Model file for the job. Use its own axes, mm. A direction names the side the tool comes from. Give positions to 0.01 mm unless a question says otherwise; leave off trailing zeros. Write each loop counter-clockwise with the first axis right and the second up, starting at its lowest first coordinate (ties: lowest second). Pieces come first, ordered by that corner, then holes.
```python
from build123d import *

# Parameters (mm, degrees)
EXTRUDE1_DEPTH          = 15.875
SKETCH2_W               = 56.3626
SKETCH2_H               = 56.3626
CUT_EXTRUDE1_DEPTH      = 3.9624
SKETCH3_W               = 56.3626
SKETCH3_H               = 56.3626
CUT_EXTRUDE2_DEPTH      = 3.9624
CUT_EXTRUDE3_DEPTH      = 174.221342401
CUT_EXTRUDE4_DEPTH      = 138.612224622
SKETCH7_R               = 3.175
CUT_EXTRUDE6_DEPTH      = 174.221342401
CUT_EXTRUDE7_DEPTH      = 3.9624
CUT_EXTRUDE7_DEPTH_BACK = 133.865789145
SKETCH9_R               = 3.175


with BuildPart() as part:
    # Sketch1 → Extrude1 (new body)
    with BuildSketch(Plane.XY):
        with BuildLine():
            Line((108.579689187, 130.408922074), (87.518897096, 109.348129983))
            ThreePointArc((87.518897096, 109.348129983), (85.973830897, 108.315749755), (84.15130105, 107.953226029))
            Line((84.15130105, 107.953226029), (61.485993141, 107.953226029))
            Line((61.485993141, 107.953226029), (57.548993141, 104.016226029))
            Line((57.548993141, 104.016226029), (57.548993141, 101.450826029))
            Line((57.548993141, 101.450826029), (62.120993141, 96.878826029))
            Line((62.120993141, 96.878826029), (104.411993141, 96.878826029))
            Line((104.411993141, 96.878826029), (108.983993141, 101.450826029))
            Line((108.983993141, 101.450826029), (108.983993141, 106.657826029))
            ThreePointArc((108.983993141, 106.657826029), (109.653547039, 108.27427213), (111.269993141, 108.943826029))
            Line((111.269993141, 108.943826029), (116.476993141, 108.943826029))
            Line((116.476993141, 108.943826029), (121.048993141, 113.515826029))
            Line((121.048993141, 113.515826029), (121.048993141, 155.806826029))
            Line((121.048993141, 155.806826029), (116.476993141, 160.378826029))
            Line((116.476993141, 160.378826029), (113.911593141, 160.378826029))
            Line((113.911593141, 160.378826029), (109.974593141, 156.441826029))
            Line((109.974593141, 156.441826029), (109.974593141, 133.776518119))
            ThreePointArc((109.974593141, 133.776518119), (109.612069415, 131.953988273), (108.579689187, 130.408922074))
        make_face()
    extrude(amount=EXTRUDE1_DEPTH)

    # Sketch2 → Cut-Extrude1 (cut)
    with BuildSketch(Plane.XY.offset(15.875)):
        with Locations((85.730293141, 132.197526029)):
            Rectangle(SKETCH2_W, SKETCH2_H)
    extrude(amount=-CUT_EXTRUDE1_DEPTH, mode=Mode.SUBTRACT)

    # Sketch3 → Cut-Extrude2 (cut)
    with BuildSketch(Plane(origin=(0, 0, 0), x_dir=(-1, 0, 0), z_dir=(0, 0, -1))):
        with Locations((-85.730293141, 132.197526029)):
            Rectangle(SKETCH3_W, SKETCH3_H)
    extrude(amount=-CUT_EXTRUDE2_DEPTH, mode=Mode.SUBTRACT)

    # Sketch4 → Cut-Extrude3 (cut, through all)
    with BuildSketch(Plane.ZY.offset(-57.548993141)):
        Polygon((0, 101.450826029), (4.572, 96.878826029), (11.303, 96.878826029), (15.875, 101.450826029), (19.712057388, 96.14079716), (9.313004955, 92.313845979), (-3.516713195, 97.866362975), align=None)
    extrude(amount=-CUT_EXTRUDE3_DEPTH, mode=Mode.SUBTRACT)

    # Sketch6 → Cut-Extrude4 (cut, through all)
    with BuildSketch(Plane(origin=(0, 160.378826029, 0), x_dir=(1, 0, 0), z_dir=(0, 1, 0))):
        Polygon((116.476993141, -15.875), (121.048993141, -11.303), (121.048993141, -4.572), (116.476993141, 0), (122.85176925, 1.025817626), (123.595758284, -16.192214298), (117.254137473, -18.459609448), align=None)
    extrude(amount=-CUT_EXTRUDE4_DEPTH, mode=Mode.SUBTRACT)

    # Sketch7 → Cut-Extrude6 (cut, through all)
    with BuildSketch(Plane.ZY.offset(-57.548993141)):
        with Locations((7.9375, 136.579026029)):
            Circle(SKETCH7_R)
        with Locations((7.9375, 152.454026029)):
            Circle(SKETCH7_R)
    extrude(amount=-CUT_EXTRUDE6_DEPTH, mode=Mode.SUBTRACT)

    # Sketch9 → Cut-Extrude7 (cut, two sides: drawn at the far end of the back side and taken through both)
    with BuildSketch(Plane(origin=(0, 107.953226029, 0), x_dir=(1, 0, 0), z_dir=(0, 1, 0)).offset(-CUT_EXTRUDE7_DEPTH_BACK)):
        with Locations(Location((65.473793141, -7.9375, 0), (0, 0, 90))):
            Circle(SKETCH9_R)
        with Locations(Location((81.348793141, -7.9375, 0), (0, 0, 28.032682271))):
            Circle(SKETCH9_R)
    extrude(amount=CUT_EXTRUDE7_DEPTH + CUT_EXTRUDE7_DEPTH_BACK, mode=Mode.SUBTRACT)


solid = part.part
```
1. Probe probe 1 along Z at (x, y) = (109, 111); probe 2 along Y at (x, z) = (111.5, 8); probe 3 along Z at (x, y) = (66.5, 103) (3 decimals). List the from-to ranges inside material, lowest first.
Calculated:
probe 1: z = 3.96 to 11.91
probe 2: y = 108.94 to 133.4, 139.75 to 149.28, 155.63 to 157.97
probe 3: z = 0 to 4.933, 10.942 to 15.875
2. Which spindle directions (+Z, -Z, +X, -X, +Y, -Y) get a long thin tool onto all of the face, cutting with end or side? Do faces 1 (the flat face through (109.975, 145, 8)), 2 (the flat face through (113.912, 134, 2)), 3 (the flat face through (108.984, 103, 8)). Say none if no direction does.
Calculated:
face 1: +Z, -Z, -X, +Y
face 2: -Z, -X, +Y, -Y
face 3: +Z, -Z, +X, -Y
3. Slice it at B-B, the plane z = 12.75. Write the cut outline in (x, y).
Calculated:
outline: (57.55, 101.45) - (60.67, 98.33) - (105.86, 98.33) - (108.98, 101.45) - (108.98, 104.02) - (57.55, 104.02) - close; (113.91, 108.94) - (116.48, 108.94) - (119.6, 112.07) - (119.6, 157.25) - (116.48, 160.38) - (113.91, 160.38) - close
4. Slice it at C-C, the plane y = 145. Write the cut outline in (x, z) (3 decimals).
Calculated:
outline: (109.975, 3.962) - (113.912, 3.962) - (113.912, 0) - (116.477, 0) - (121.049, 4.572) - (121.049, 11.303) - (116.477, 15.875) - (113.912, 15.875) - (113.912, 11.913) - (109.975, 11.913) - close
5. Slice it at D-D, the plane x = 77. Write the cut outline in (y, z) (3 decimals).
Calculated:
outline: (96.879, 4.572) - (101.451, 0) - (104.016, 0) - (104.016, 3.962) - (107.953, 3.962) - (107.953, 11.913) - (104.016, 11.913) - (104.016, 15.875) - (101.451, 15.875) - (96.879, 11.303) - close
6. Pin check, flat tips, straight feed: P1, Ø4, axis at x = 113, z = 9, coming from the -Y side; P2, Ø2, axis at x = 109.5, z = 14, coming from the -Y side; P3, Ø3, axis at y = 138, z = 13.5, coming from the -X side; P4, Ø6, axis at y = 131, z = 11.5, coming from the +X side. Stop position of each tip, or through.
Calculated:
P1: stops at y = 108.93
P2: stops at y = 100.97
P3: stops at x = 113.91
P4: stops at x = 121.05
7. Slice it at A-A, the plane z = 8.25. State how many separate pieces and enclosed holes the cut face has, and give its area (3 significant figures).
Calculated:
separate pieces: 5
enclosed holes: 0
area: 1,090 mm2
8. Pull direction X, two halves, no side cores. Call faces 4 (the cylindrical face through (109.64, 108.26, 7.88)), 5 (the flat face through (111.97, 158.44, 7.88)), 6 (the cylindrical face through (62.326, 102.339, 8.351)), 7 (the cylindrical face through (115.427, 139.727, 7.524)): +X half, -X half, draft (parallel to the pull), parting line (faces both ways), or undercut.
Calculated:
face 4: +X half
face 5: -X half
face 6: undercut
face 7: draft
